```python
from build123d import *

# Parameters (mm, degrees)
BOSS_EXTRUDE1_DEPTH = 10
FILLET1_R           = 1


with BuildPart() as part:
    # Sketch1 → Boss-Extrude1 (new body)
    with BuildSketch(Plane.XY):
        with BuildLine():
            Line((0, 1.049183312), (0, -1.049183312))
            ThreePointArc((0, -1.049183312), (-0.161869295, -1.594652762), (-0.595073842, -1.963532701))
            Line((-0.595073842, -1.963532701), (-3.306595396, -3.16434939))
            ThreePointArc((-3.306595396, -3.16434939), (-3.504578796, -3.228353052), (-3.711521554, -3.25))
            Line((-3.711521554, -3.25), (-27.169029734, -3.25))
            ThreePointArc((-27.169029734, -3.25), (-27.199985158, -3.249520766), (-27.230910912, -3.248083523))
            Line((-27.230910912, -3.248083523), (-51.261881178, -1.758163367))
            ThreePointArc((-51.261881178, -1.758163367), (-51.928656702, -1.444958965), (-52.2, -0.760079844))
            Line((-52.2, -0.760079844), (-52.2, 0.760079844))
            ThreePointArc((-52.2, 0.760079844), (-51.928656702, 1.444958965), (-51.261881178, 1.758163367))
            Line((-51.261881178, 1.758163367), (-27.230910912, 3.248083523))
            ThreePointArc((-27.230910912, 3.248083523), (-27.199985158, 3.249520766), (-27.169029734, 3.25))
            Line((-27.169029734, 3.25), (-3.711521554, 3.25))
            ThreePointArc((-3.711521554, 3.25), (-3.504578796, 3.228353052), (-3.306595396, 3.16434939))
            Line((-3.306595396, 3.16434939), (-0.595073842, 1.963532701))
            ThreePointArc((-0.595073842, 1.963532701), (-0.161869295, 1.594652762), (0, 1.049183312))
        make_face()
    extrude(amount=BOSS_EXTRUDE1_DEPTH)

    # Fillet1
    fillet1_edges = [part.edges().sort_by_distance(p)[0] for p in [
        (-3.504578796, -3.228353052, 10),
        (-1.950834619, -2.563941045, 10),
        (-39.246396045, -2.503123445, 0),
        (-51.928656702, -1.444958965, 0),
        (-52.2, 0, 0),
        (-51.928656702, 1.444958965, 0),
        (-39.246396045, 2.503123445, 0),
        (-0.161869295, -1.594652762, 10),
        (-27.199985158, 3.249520766, 0),
        (-15.440275644, 3.25, 0),
        (-3.504578796, 3.228353052, 0),
        (-1.950834619, 2.563941045, 0),
        (-0.161869295, 1.594652762, 0),
        (0, 0, 0),
        (-0.161869295, -1.594652762, 0),
        (-1.950834619, -2.563941045, 0),
        (0, 0, 10),
        (-3.504578796, -3.228353052, 0),
        (-15.440275644, -3.25, 0),
        (-27.199985158, -3.249520766, 0),
        (-0.161869295, 1.594652762, 10),
        (-1.950834619, 2.563941045, 10),
        (-3.504578796, 3.228353052, 10),
        (-15.440275644, 3.25, 10),
        (-27.199985158, 3.249520766, 10),
        (-39.246396045, 2.503123445, 10),
        (-27.199985158, -3.249520766, 10),
        (-51.928656702, 1.444958965, 10),
        (-52.2, 0, 10),
        (-51.928656702, -1.444958965, 10),
        (-39.246396045, -2.503123445, 10),
        (-15.440275644, -3.25, 10),
    ]]
    fillet(fillet1_edges, radius=FILLET1_R)


solid = part.part
```
Input: part model. Units: mm. Frame: model coordinates. Round coordinates to 2 decimals unless told otherwise and drop trailing zeros. Write each loop counter-clockwise with the first axis right and the second up, starting at its lowest first coordinate (ties: lowest second). Pieces come first, ordered by that corner, then holes. Notation, with made-up numbers: (-25.5, 87.25) -> (22.5, 87.25) arc R17 ccw to (22.5, 115.25) -> close; hole circle Ø8 at (69, -34.75). An arc over 180 degrees is marked (long way). Answer as CSV lines item,"result".
1. Mould query, pull axis X, two halves, no side actions, for faces 1 (the flat face through (-20, 0, 0)), 2 (the cylindrical face through (-51.936, 1.437, 4.944)), 3 (the flat face through (0, 0, 5)). Classes: +X half, -X half, draft (parallel to the pull), parting line (faces both ways), or undercut.
Geometry says:
face 1,"draft"
face 2,"-X half"
face 3,"+X half"
2. Ray query, L1, parallel to Y at x = -28, z = 3; L2, parallel to X at y = 1, z = 8.5; L3, parallel to Z at x = -38.5, y = -2. Return the intervals inside material, ascending. Write a range as [from, to].
Geometry says:
L1,"y = [-3.2, 3.2]"
L2,"x = [-52.17, 0]"
L3,"z = [0.11, 9.89]"
3. Section A-A (z = 2.25). Return the cut outline in (x, y).
Geometry says:
outline,"(-52.2, -0.76) arc R1 ccw to (-51.26, -1.76) -> (-27.23, -3.25) arc R1 ccw to (-27.17, -3.25) -> (-3.71, -3.25) arc R1 ccw to (-3.31, -3.16) -> (-0.6, -1.96) arc R1 ccw to (0, -1.05) -> (0, 1.05) arc R1 ccw to (-0.6, 1.96) -> (-3.31, 3.16) arc R1 ccw to (-3.71, 3.25) -> (-27.17, 3.25) arc R1 ccw to (-27.23, 3.25) -> (-51.26, 1.76) arc R1 ccw to (-52.2, 0.76) -> close"
4. Contact query for flat-ended pins moving along their axis: P1, Ø3, axis at y = 1.5, z = 5, coming from the -X side; P2, Ø2, axis at y = 2.5, z = 6.5, coming from the -X side. Output: stop coordinate, or through.
Geometry says:
P1,"stops at x = -52.2"
P2,"stops at x = -51.87"
